The listing builds one solid part. Answer for the finished solid, in the listing's coordinates (mm). Give positions to 0.01 mm unless a question says otherwise; leave off trailing zeros. Loops run counter-clockwise (first coordinate to the right, second up) from the corner with the lowest first, then second, coordinate; pieces in that order, holes last. Notation, with made-up numbers: (-1, 56) - (58, 56) arc R19 ccw to (58, 73) - close; hole circle Ø11 at (-15, 51.5). An arc over 180 degrees is marked (long way). Answer in a Markdown table with one row per item. Add a question column.
```python
from build123d import *

# Parameters (mm, degrees)
SKETCH1_R           = 5
BOSS_EXTRUDE1_DEPTH = 115
SKETCH2_R           = 1.5
BOSS_EXTRUDE2_DEPTH = 1
SKETCH3_R           = 0.5
BOSS_EXTRUDE3_DEPTH = 0.5
SKETCH4_R           = 3.63725935
SKETCH4_R_2         = 3.411929034
CUT_EXTRUDE1_DEPTH  = 0.5
FILLET1_R           = 1
FILLET2_R           = 1
FILLET6_R           = 0.55
FILLET7_R           = 0.1


with BuildPart() as part:
    # Sketch1 → Boss-Extrude1 (new body)
    with BuildSketch(Plane(origin=(0, 0, 0), x_dir=(1, 0, 0), z_dir=(0, 1, 0))):
        with Locations(Location((0, 0, 0), (0, 0, 270))):
            Circle(SKETCH1_R)
    extrude(amount=BOSS_EXTRUDE1_DEPTH)

    # Sketch2 → Boss-Extrude2 (add)
    with BuildSketch(Plane.XZ):
        with Locations(Location((0, 0, 0), (0, 0, 90))):
            Circle(SKETCH2_R)
    extrude(amount=BOSS_EXTRUDE2_DEPTH)

    # Sketch3 → Boss-Extrude3 (add)
    with BuildSketch(Plane.XZ.offset(1)):
        with Locations(Location((0, 0, 0), (0, 0, 270))):
            Circle(SKETCH3_R)
    extrude(amount=BOSS_EXTRUDE3_DEPTH)

    # Sketch4 → Cut-Extrude1 (cut)
    with BuildSketch(Plane(origin=(0, 115, 0), x_dir=(1, 0, 0), z_dir=(0, 1, 0))):
        with Locations(Location((0, 0, 0), (0, 0, 270))):
            Circle(SKETCH4_R)
        with Locations(Location((0, 0, 0), (0, 0, 270))):
            Circle(SKETCH4_R_2, mode=Mode.SUBTRACT)
    extrude(amount=-CUT_EXTRUDE1_DEPTH, mode=Mode.SUBTRACT)

    # Fillet1
    # the kernel refuses this fillet: 1 mm, written as the material it takes off along each edge
    with BuildSketch(Plane(origin=(0, 115, 0), x_dir=(0, 0, 1), z_dir=(-1, 0, 0))) as fillet1_piece_1:
        with BuildLine():
            CenterArc((4.503284754, -1), FILLET1_R, 90, 60)
            Line((3.63725935, -0.5), (3.619938842, -0.49))
            ThreePointArc((3.619938842, -0.49), (3.61725935, -0.25), (3.61725935, 0))
            Line((3.61725935, 0), (3.63725935, 0.02))
            Line((3.63725935, 0.02), (4.503284754, 0.02))
            Line((4.503284754, 0.02), (4.503284754, 0))
        make_face()
    revolve(axis=Axis((0, 115, 0), (0, 1, 0)), mode=Mode.SUBTRACT)
    with BuildSketch(Plane(origin=(0, 115, 0), x_dir=(0, 0, 1), z_dir=(-1, 0, 0))) as fillet1_piece_2:
        with BuildLine():
            CenterArc((2.545903631, -1), FILLET1_R, 30, 60)
            Line((2.545903631, 0), (2.545903631, 0.02))
            Line((2.545903631, 0.02), (3.411929034, 0.02))
            Line((3.411929034, 0.02), (3.431929034, 0))
            ThreePointArc((3.431929034, 0), (3.431929034, -0.25), (3.429249543, -0.49))
            Line((3.429249543, -0.49), (3.411929034, -0.5))
        make_face()
    revolve(axis=Axis((0, 115, 0), (0, 1, 0)), mode=Mode.SUBTRACT)

    # Fillet2
    fillet2_edges = [part.edges().sort_by_distance(p)[0] for p in [
        (0, 0, -5),
    ]]
    fillet(fillet2_edges, radius=FILLET2_R)

    # Fillet6
    fillet6_edges = [part.edges().sort_by_distance(p)[0] for p in [
        (0, -1, -1.5),
    ]]
    fillet(fillet6_edges, radius=FILLET6_R)

    # Fillet7
    fillet7_edges = [part.edges().sort_by_distance(p)[0] for p in [
        (0, -1.5, 0.5),
    ]]
    fillet(fillet7_edges, radius=FILLET7_R)


solid = part.part
```
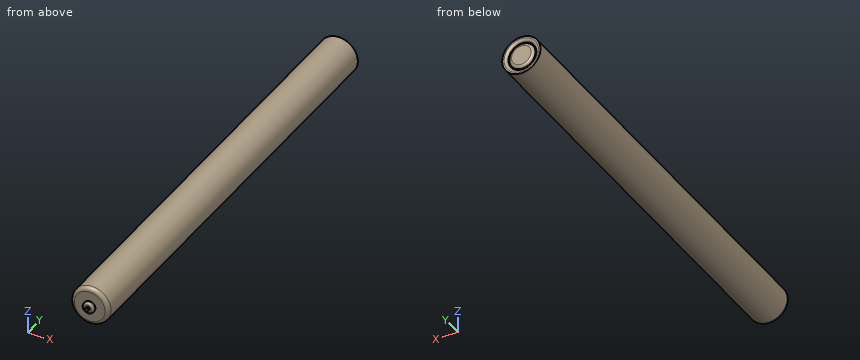
(1) Given pin 1 Ø3 at (x, y) = (2, 78.5) entering from +Z; pin 2 Ø1.5 at (x, z) = (2, -3.5) entering from -Y; pin 3 Ø1 at (x, y) = (-3.5, 92.5) entering from +Z, each flat-ended and moving along its own axis, determine where each tip first touches the part or whether it passes through.
(2) Find the intervals of material crossed by line 1 along Y through (x, z) = (0, 2); line 2 along Y through (x, z) = (-0.75, 4.75); line 3 along X through (y, z) = (97.5, 3), in increasing order. Write a range as [from, to].
(3) A cutting plane is placed at A-A on y = 79. Determine the outline of the cut face in (x, z).
Evaluation:
| question | item | result |
|---|---|---|
| 1 | pin 1 | stops at z = 4.97 |
| 1 | pin 2 | stops at y = 0 |
| 1 | pin 3 | stops at z = 4 |
| 2 | line 1 | y = [0, 115] |
| 2 | line 2 | y = [0.41, 115] |
| 2 | line 3 | x = [-4, 4] |
| 3 | outline | circle Ø10 at (0, 0) |
